Read the model definition and answer for the solid it produces. Units are mm, in the model's axes. Face numbers are marked on the shaded views. A direction names the side the tool comes from. Coordinates: 2 decimals unless noted, no trailing zeros. Order: outer loops, then holes, each group sorted by start corner. A loop starts at its lowest first (then second) coordinate and runs counter-clockwise, first axis right, second up.
from build123d import *

# Parameters (mm, degrees)
F1_DEPTH = 25
F3_R     = 2


with BuildPart() as f1:
    # F0 (on Top) → F1 (new body)
    with BuildSketch(Plane.XY):
        Polygon((20, 2), (23, 2), (23, 10), (-5, 10), (-5, 0), (0, 0), (0, 5), (20, 5), align=None)
    extrude(amount=F1_DEPTH)

    # F2: F1 across plane


with BuildPart() as f1_1:
    add(f1.part)
    add(f1.part.mirror(Plane.XZ))

    # F3
    f3_edges = [f1_1.edges().sort_by_distance(p)[0] for p in [
        (0, 5, 12.5),
        (0, -5, 12.5),
        (23, 2, 12.5),
        (23, -2, 12.5),
        (-5, 0, 25),
        (-5, 0, 0),
        (23, 6, 25),
        (23, -6, 25),
        (23, -6, 0),
        (23, 6, 0),
    ]]
    fillet(f3_edges, radius=F3_R)


solid = f1_1.part
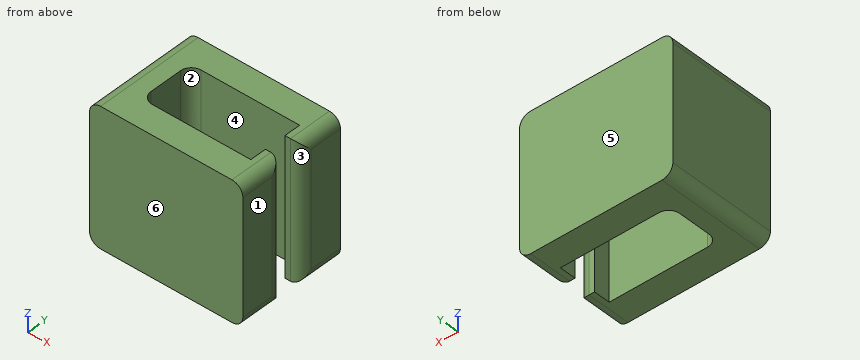
Q1. The part is cut by section C-C, the plane y = -4.5. Determine the outline of the cut face in (x, z).
Q2. The part is cut by section B-B, the plane z = 21.25. Determine the outline of the cut face in (x, y), then the cut area to 3 significant figures.
Q3. Which of the six approach directions +Z, -Z, +X, -X, +Y, -Y give full straight-line access (tool end or side, diameter ignored) to the marked faces 1, 2 and 3?
Q4. The part is cut by section A-A, the plane x = 5.5. Determine the outline of the cut face in (y, z).
Q5. Straight lines are drawn through the part: L1, parallel to Y at x = 2.75, z = 15; L2, parallel to Y at x = 21, z = 13.5; L3, parallel to X at y = 2.75, z = 19.75. For each, find the intervals that lie inside material, in ascending order.
Q6. Each of these flat-tipped pins is pushed along its axis until it touches: P1, Ø12, axis at y = 1.5, z = 4.5, coming from the +X side; P2, Ø3, axis at y = -1.5, z = 18, coming from the +X side; P3, Ø1.5, axis at y = 0, z = 12.5, coming from the +X side. Where does it stop, or does it pass through?
Q7. Determine the mould class of the marked faces 4, 5 and 6 for opening direction Y: +Y half, -Y half, draft (parallel to the pull), parting line (faces both ways), or undercut.
Q8. The part is cut by section D-D, the plane y = 1.5. Determine the outline of the cut face in (x, z).
Computed values:
1. outline: (-5, 2) arc R2 ccw to (-3, 0) - (0.68, 0) - (0.68, 25) - (-3, 25) arc R2 ccw to (-5, 23) - close; (20, 0) - (21, 0) arc R2 ccw to (23, 2) - (23, 23) arc R2 ccw to (21, 25) - (20, 25) - close
2. outline: (-5, -10) - (23, -10) - (23, -4) arc R2 ccw to (21, -2) - (20, -2) - (20, -5) - (2, -5) arc R2 cw to (0, -3) - (0, 3) arc R2 cw to (2, 5) - (20, 5) - (20, 2) - (21, 2) arc R2 ccw to (23, 4) - (23, 10) - (-5, 10) - close
2. area: 348 mm2
3. face 1: +Z, -Z, +X, +Y, -Y
3. face 2: +Z, -Z
3. face 3: +Z, -Z, +X
4. outline: (-10, 0) - (-5, 0) - (-5, 25) - (-10, 25) - close; (5, 0) - (10, 0) - (10, 25) - (5, 25) - close
5. L1: y = -10 to -5, 5 to 10
5. L2: y = -10 to -2, 2 to 10
5. L3: x = -5 to 0, 20 to 22.56
6. P1: stops at x = 23
6. P2: stops at x = 22.73
6. P3: stops at x = 0
7. face 4: undercut
7. face 5: +Y half
7. face 6: -Y half
8. outline: (-5, 2) arc R2 ccw to (-3, 0) - (0, 0) - (0, 25) - (-3, 25) arc R2 ccw to (-5, 23) - close
